Can you work these out from the model? Positions are in its coordinate system, mm. Face numbers are marked on the shaded views. A direction names the side the tool comes from. Give positions to 0.01 mm unless a question says otherwise; leave off trailing zeros. Order: outer loops, then holes, each group sorted by start corner. A loop starts at its lowest first (then second) coordinate and runs counter-clockwise, first axis right, second up. Notation, with made-up numbers: M 25.25,57.5 L 84.25,57.5 A21 cw 84.25,89.5 Z; hole C 70.5,80.25 d7. An arc over 180 degrees is marked long. Use a Markdown table: item, result. Add a question column.
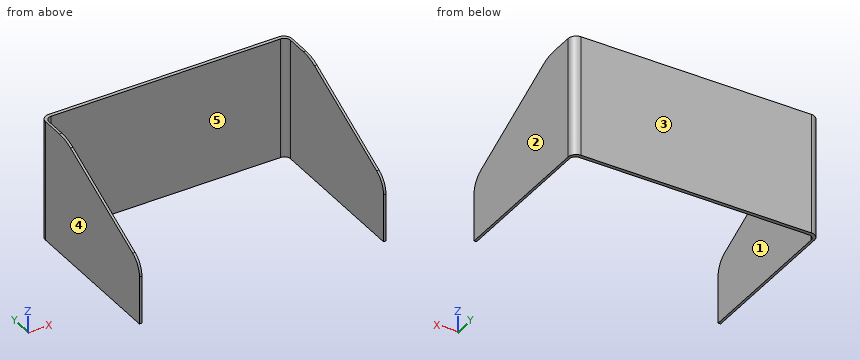
from build123d import *

# Parameters (mm, degrees)
F1_DEPTH = 60
F2_SIZE2 = 30
F2_SIZE  = 60
F3_R     = 20
F4_R     = 10
F5_R     = 3
F6_R     = 4


with BuildPart() as f1:
    # F0 (on Top) → F1 (new body)
    with BuildSketch(Plane.XY):
        Polygon((-69.0494580577, 36.7513514241), (-69.0494580577, -43.2486485759), (-67.8494580577, -43.2486485759), (-67.8494580577, 34.9513514241), (52.1505419423, 34.9513514241), (52.1505419423, -43.2486485759), (53.3505419423, -43.2486485759), (53.3505419423, 36.7513514241), align=None)
    extrude(amount=F1_DEPTH)

    # F2
    f2_edges = [f1.edges().sort_by_distance(p)[0] for p in [
        (-68.449458, -43.248649, 60),
        (52.750542, -43.248649, 60),
    ]]
    f2_side = f1.faces().sort_by_distance((-68.903233, -3.248649, 60))[0]
    chamfer(f2_edges, length=F2_SIZE, length2=F2_SIZE2, reference=f2_side)

    # F3
    f3_edges = [f1.edges().sort_by_distance(p)[0] for p in [
        (-68.449458, 16.751351, 60),
        (52.750542, 16.751351, 60),
    ]]
    fillet(f3_edges, radius=F3_R)

    # F4
    f4_edges = [f1.edges().sort_by_distance(p)[0] for p in [
        (-68.449458, -43.248649, 30),
        (52.750542, -43.248649, 30),
    ]]
    fillet(f4_edges, radius=F4_R)

    # F5
    f5_edges = [f1.edges().sort_by_distance(p)[0] for p in [
        (-67.849458, 34.951351, 30),
        (52.150542, 34.951351, 30),
    ]]
    fillet(f5_edges, radius=F5_R)

    # F6
    f6_edges = [f1.edges().sort_by_distance(p)[0] for p in [
        (53.350542, 36.751351, 30),
        (-69.049458, 36.751351, 30),
    ]]
    fillet(f6_edges, radius=F6_R)


solid = f1.part
1. If we section it at C-C, the plane x = -18: List the corners of the cut face in (y, z) for me, then the cut area to 3 significant figures.
2. If we section it at D-D, the plane y = -10.5: List the corners of the cut face in (x, z) for me, then the cut area to 3 significant figures.
3. I need wall thicknesses on L1, parallel to X at y = -35, z = 10; L2, parallel to Y at x = 1.5, z = 21. Which ranges of each line are inside material? Lowest first, please. Write a range as [from, to].
4. If we section it at A-A, the plane y = -21: List the corners of the cut face in (x, z) for me, then the cut area to 3 significant figures.
5. We'd pull the mould along X, two halves only. Please class the marked faces 1, 2 and 3: +X half, -X half, draft (parallel to the pull), parting line (faces both ways), or undercut.
6. If we section it at B-B, the plane z = 22.5: List the corners of the cut face in (x, y) for me.
7. On a 3-axis mill with a long thin cutter (end or side, diameter ignored), from which of +Z, -Z, +X, -X, +Y, -Y can I reach the whole of each face in a straight line? I mean the marked faces 4 and 5. Say none if no direction works.
8. Will this pin go through, and if not, where does the flat tip stop? pin 1 (3 mm diameter, centred on x = 15.5, z = 35.5, fed in from -Y).
Geometry results:
| question | item | result |
|---|---|---|
| 1 | outline | M 34.95,0 L 36.75,0 L 36.75,60 L 34.95,60 Z |
| 1 | area | 108 mm^2 |
| 2 | outline | M -69.05,0 L -67.85,0 L -67.85,46.37 L -69.05,46.37 Z; M 52.15,0 L 53.35,0 L 53.35,46.37 L 52.15,46.37 Z |
| 2 | area | 111 mm^2 |
| 3 | L1 | x = [-69.05, -67.85], [52.15, 53.35] |
| 3 | L2 | y = [34.95, 36.75] |
| 4 | outline | M -69.05,0 L -67.85,0 L -67.85,41.12 L -69.05,41.12 Z; M 52.15,0 L 53.35,0 L 53.35,41.12 L 52.15,41.12 Z |
| 4 | area | 98.7 mm^2 |
| 5 | face 1 | undercut |
| 5 | face 2 | +X half |
| 5 | face 3 | draft |
| 6 | outline | M -69.05,-43.25 L -67.85,-43.25 L -67.85,31.95 A3 cw -64.85,34.95 L 49.15,34.95 A3 cw 52.15,31.95 L 52.15,-43.25 L 53.35,-43.25 L 53.35,32.75 A4 ccw 49.35,36.75 L -65.05,36.75 A4 ccw -69.05,32.75 Z |
| 7 | face 4 | +Z, -Z, -X, +Y, -Y |
| 7 | face 5 | +Z, -Z, -Y |
| 8 | pin 1 | stops at y = 34.95 |
